```python
from build123d import *

# Parameters (mm, degrees)
SKETCH_1_W               = 35
SKETCH_1_H               = 26
SKETCH_1_R               = 2.25
EXTRUDE_1_DEPTH          = 6
CUT_EXTRUDE_1_DEPTH      = 23.610838109
CUT_EXTRUDE_1_DEPTH_BACK = 23.610838109
SKETCH_3_R               = 1.05


with BuildPart() as part:
    # 草图1 → 凸台-拉伸1 (new body)
    with BuildSketch(Plane(origin=(0, 0, 0), x_dir=(1, 0, 0), z_dir=(0, 1, 0))):
        Rectangle(SKETCH_1_W, SKETCH_1_H)
        with Locations(Location((-12.5, 8, 0), (0, 0, 270))):
            Circle(SKETCH_1_R, mode=Mode.SUBTRACT)
        with Locations(Location((12.5, 8, 0), (0, 0, 90))):
            Circle(SKETCH_1_R, mode=Mode.SUBTRACT)
        with Locations(Location((-12.5, -8, 0), (0, 0, 90))):
            Circle(SKETCH_1_R, mode=Mode.SUBTRACT)
        with Locations(Location((12.5, -8, 0), (0, 0, 270))):
            Circle(SKETCH_1_R, mode=Mode.SUBTRACT)
    extrude(amount=EXTRUDE_1_DEPTH)

    # 草图3 → 切除-拉伸1 (cut, two sides: drawn at the far end of the back side and taken through both)
    with BuildSketch(Plane.XY.offset(-CUT_EXTRUDE_1_DEPTH_BACK)):
        with Locations((0, 6)):
            Circle(SKETCH_3_R)
        with Locations((5, 6)):
            Circle(SKETCH_3_R)
        with Locations((10, 6)):
            Circle(SKETCH_3_R)
        with Locations((15, 6)):
            Circle(SKETCH_3_R)
        with Locations((-5, 6)):
            Circle(SKETCH_3_R)
        with Locations((-10, 6)):
            Circle(SKETCH_3_R)
        with Locations((-15, 6)):
            Circle(SKETCH_3_R)
    extrude(amount=CUT_EXTRUDE_1_DEPTH + CUT_EXTRUDE_1_DEPTH_BACK, mode=Mode.SUBTRACT)


solid = part.part
```
Can you work these out from the model? Positions are in its coordinate system, mm. Give positions to 0.01 mm unless a question says otherwise; leave off trailing zeros. Write each loop counter-clockwise with the first axis right and the second up, starting at its lowest first coordinate (ties: lowest second). Pieces come first, ordered by that corner, then holes. Notation, with made-up numbers: (53.25, -23) -> (90.25, -23) arc R24 cw to (90.25, 12) -> close; hole circle Ø7 at (42, 51). An arc over 180 degrees is marked (long way). One line per item, written item: value.
Q1. Imagine slicing it at B-B on z = -7. Please give me the cut outline in (x, y), and give its area (3 significant figures).
Results found:
outline: (-17.5, 0) -> (-14.52, 0) -> (-14.52, 5.07) arc R1.05 cw to (-16.05, 6) -> (-17.5, 6) -> close; (-10.48, 0) -> (10.48, 0) -> (10.48, 5.07) arc R1.05 cw to (8.95, 6) -> (6.05, 6) arc R1.05 cw to (3.95, 6) -> (1.05, 6) arc R1.05 cw to (-1.05, 6) -> (-3.95, 6) arc R1.05 cw to (-6.05, 6) -> (-8.95, 6) arc R1.05 cw to (-10.48, 5.07) -> close; (14.52, 0) -> (17.5, 0) -> (17.5, 6) -> (16.05, 6) arc R1.05 cw to (14.52, 5.07) -> close
area: 151 mm^2
Q2. For P1, Ø3.5, axis at x = 12.5, z = 8, coming from the -Y side, with a flat end and sliding along its axis, tell me the tip position at first contact or that it passes through.
Results found:
P1: passes through
Q3. Please list where these lines run through material, in increasing order: line 1 (Z direction, x = -12.5, y = 1.75); line 2 (X direction, y = 3.25, z = 8); line 3 (X direction, y = 3.75, z = 8.75). Write a range as [from, to].
Results found:
line 1: z = [-13, -10.25], [-5.75, 5.75], [10.25, 13]
line 2: x = [-17.5, -14.75], [-10.25, 10.25], [14.75, 17.5]
line 3: x = [-17.5, -14.62], [-10.38, 10.38], [14.62, 17.5]
Q4. We'd pull the mould along Z, two halves only. Please class faces 1 (the face through (17, 6, 0)), 2 (the face through (-14.696, 2.958, -8.488)), 3 (the face through (-10.304, 2.958, 8.488)), 4 (the face through (0, 3, 13)): +Z half, -Z half, draft (parallel to the pull), parting line (faces both ways), or undercut.
Results found:
face 1: draft
face 2: undercut
face 3: undercut
face 4: +Z half
Q5. Imagine slicing it at D-D on z = 2. Please give me the cut outline in (x, y).
Results found:
outline: (-17.5, 0) -> (17.5, 0) -> (17.5, 6) -> (16.05, 6) arc R1.05 cw to (13.95, 6) -> (11.05, 6) arc R1.05 cw to (8.95, 6) -> (6.05, 6) arc R1.05 cw to (3.95, 6) -> (1.05, 6) arc R1.05 cw to (-1.05, 6) -> (-3.95, 6) arc R1.05 cw to (-6.05, 6) -> (-8.95, 6) arc R1.05 cw to (-11.05, 6) -> (-13.95, 6) arc R1.05 cw to (-16.05, 6) -> (-17.5, 6) -> close
Q6. Imagine slicing it at C-C on x = 11.5. Please give me the cut outline in (y, z).
Results found:
outline: (0, -13) -> (6, -13) -> (6, -10.02) -> (0, -10.02) -> close; (0, -5.98) -> (6, -5.98) -> (6, 5.98) -> (0, 5.98) -> close; (0, 10.02) -> (6, 10.02) -> (6, 13) -> (0, 13) -> close
Q7. Imagine slicing it at A-A on y = 3.75. Please give me the cut outline in (x, z), and give its area (3 significant figures).
Results found:
outline: (-17.5, -13) -> (17.5, -13) -> (17.5, 13) -> (-17.5, 13) -> close; hole circle Ø4.5 at (-12.5, -8); hole circle Ø4.5 at (-12.5, 8); hole circle Ø4.5 at (12.5, -8); hole circle Ø4.5 at (12.5, 8)
area: 846 mm^2
